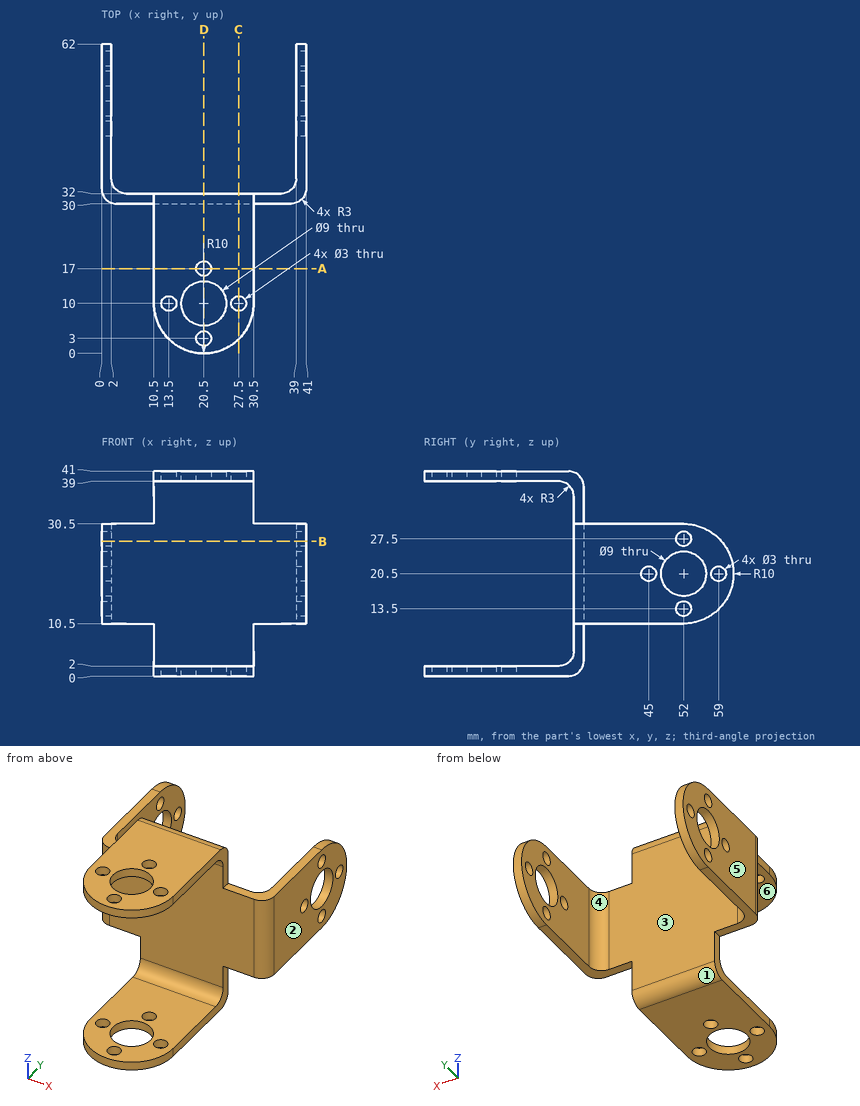
Can you work these out from the drawing? Everything is in mm from the part's minimum corner. A direction names the side the tool comes from. Give positions to 0.01 mm unless a question says otherwise; leave off trailing zeros. Loops run counter-clockwise (first coordinate to the right, second up) from the corner with the lowest first, then second, coordinate; pieces in that order, holes last. Notation, with made-up numbers: (4.25, 68.5) -> (31.25, 68.5) arc R31 ccw to (31.25, 103.5) -> close; hole circle Ø3 at (-9.75, 1). An arc over 180 degrees is marked (long way). Return JSON: item names as keys, results as strings.
Q1. On a 3-axis mill with a long thin cutter (end or side, diameter ignored), from which of +Z, -Z, +X, -X, +Y, -Y can I reach the whole of each face in a straight line? I mean the marked faces 4, 5 and 6. Say none if no direction works.
Checks:
{"face 4": "+Z, -Z, +Y", "face 5": "+Z, -Z, -X, +Y, -Y", "face 6": "+X, -X, -Y"}
Q2. For pin 1 Ø5 at (x, z) = (12, 19) entering from +Y; pin 2 Ø11.5 at (y, z) = (23, 36) entering from -X; pin 3 Ø5 at (x, y) = (3.5, 42.5) entering from +Z, each with a flat end and sliding along its axis, tell me the tip position at first contact or that it passes through.
Checks:
{"pin 1": "stops at y = 32", "pin 2": "stops at x = 10.5", "pin 3": "stops at z = 30.5"}
Q3. I want a section at C-C, the plane x = 27.5. List the corners of the cut face in (y, z) for me, then the cut area to 3 significant figures.
Checks:
{"outline": "(2.86, 0) -> (8.5, 0) -> (8.5, 2) -> (2.86, 2) -> close; (2.86, 39) -> (8.5, 39) -> (8.5, 41) -> (2.86, 41) -> close; (11.5, 0) -> (29, 0) arc R3 ccw to (32, 3) -> (32, 38) arc R3 ccw to (29, 41) -> (11.5, 41) -> (11.5, 39) -> (27, 39) arc R3 cw to (30, 36) -> (30, 5) arc R3 cw to (27, 2) -> (11.5, 2) -> close", "area": "179 mm2"}
Q4. I need wall thicknesses on probe 1 along X at (y, z) = (44.5, 16); probe 2 along Y at (x, z) = (20.5, 1.1); probe 3 along Y at (x, z) = (40, 20). Which ranges of each line are inside material? Lowest first, please.
Checks:
{"probe 1": "x = 0 to 2, 39 to 41", "probe 2": "y = 0 to 1.5, 4.5 to 5.5, 14.5 to 15.5, 18.5 to 31.32", "probe 3": "y = 30.76 to 43.59, 46.41 to 47.53, 56.47 to 57.59, 60.41 to 61.99"}
Q5. I want a section at A-A, the plane y = 17. List the corners of the cut face in (x, z) for me, then the cut area to 3 significant figures.
Checks:
{"outline": "(10.5, 0) -> (19, 0) -> (19, 2) -> (10.5, 2) -> close; (10.5, 39) -> (19, 39) -> (19, 41) -> (10.5, 41) -> close; (22, 0) -> (30.5, 0) -> (30.5, 2) -> (22, 2) -> close; (22, 39) -> (30.5, 39) -> (30.5, 41) -> (22, 41) -> close", "area": "68.0 mm2"}
Q6. I want a section at D-D, the plane x = 20.5. Count the separate pieces of the cut face and the enclosed holes in it, then the cut area to 3 significant figures.
Checks:
{"separate pieces": "7", "enclosed holes": "0", "area": "142 mm2"}
Q7. We'd pull the mould along X, two halves only. Please class the marked faces 1, 2 and 3: released by +X, released by -X, zero draft, split by the parting line, or undercut.
Checks:
{"face 1": "zero draft", "face 2": "released by +X", "face 3": "undercut"}
Q8. I want a section at B-B, the plane z = 27. List the corners of the cut face in (x, y) for me, then the cut area to 3 significant figures.
Checks:
{"outline": "(0, 33) arc R3 ccw to (3, 30) -> (38, 30) arc R3 ccw to (41, 33) -> (41, 50.59) -> (39, 50.59) -> (39, 35) arc R3 cw to (36, 32) -> (5, 32) arc R3 cw to (2, 35) -> (2, 50.59) -> (0, 50.59) -> close; (0, 53.41) -> (2, 53.41) -> (2, 59.6) -> (0, 59.6) -> close; (39, 53.41) -> (41, 53.41) -> (41, 59.6) -> (39, 59.6) -> close", "area": "181 mm2"}
